from build123d import *

# Parameters (mm, degrees)
F1_DEPTH = 25
F3_DEPTH = 20


with BuildPart() as f1:
    # F0 (on Top) → F1 (new body)
    with BuildSketch(Plane.XY):
        with BuildLine():
            Line((-45.816002, -33.782002), (45.816002, -33.782002))
            ThreePointArc((45.816002, -33.782002), (50.058642, -32.024642), (51.816002, -27.782002))
            Line((51.816002, -27.782002), (51.816002, 27.782002))
            ThreePointArc((51.816002, 27.782002), (50.058642, 32.024642), (45.816002, 33.782002))
            Line((45.816002, 33.782002), (-45.816002, 33.782002))
            ThreePointArc((-45.816002, 33.782002), (-50.058642, 32.024642), (-51.816002, 27.782002))
            Line((-51.816002, 27.782002), (-51.816002, -27.782002))
            ThreePointArc((-51.816002, -27.782002), (-50.058642, -32.024642), (-45.816002, -33.782002))
        make_face()
    extrude(amount=F1_DEPTH)

    # F2 (on face) → F3 (cut)
    with BuildSketch(Plane.XY.offset(25)):
        with BuildLine():
            ThreePointArc((45.816002, -31.782002), (48.644429, -30.610429), (49.816002, -27.782002))
            Line((49.816002, -27.782002), (49.816002, 27.782002))
            ThreePointArc((49.816002, 27.782002), (48.644429, 30.610429), (45.816002, 31.782002))
            Line((45.816002, 31.782002), (-45.816002, 31.782002))
            ThreePointArc((-45.816002, 31.782002), (-48.644429, 30.610429), (-49.816002, 27.782002))
            Line((-49.816002, 27.782002), (-49.816002, -27.782002))
            ThreePointArc((-49.816002, -27.782002), (-48.644429, -30.610429), (-45.816002, -31.782002))
            Line((-45.816002, -31.782002), (45.816002, -31.782002))
        make_face()
    extrude(amount=-F3_DEPTH, mode=Mode.SUBTRACT)


solid = f1.part
Part model, mm, in its own coordinate system. A direction names the side the tool comes from. Round coordinates to 2 decimals unless told otherwise and drop trailing zeros. Loops run counter-clockwise (first coordinate to the right, second up) from the corner with the lowest first, then second, coordinate; pieces in that order, holes last. Notation, with made-up numbers: (-31.5, 60) - (-3.5, 60) arc R19 ccw to (-3.5, 78) - close; hole circle Ø7 at (47.5, 30.5). An arc over 180 degrees is marked (long way). Answer as a JSON object with one key per item and string values.
Item 1: Wall check: L1, parallel to X at y = 18, z = 11; L2, parallel to Y at x = 18, z = 22; L3, parallel to Z at x = 36, y = -14. Give the ranges that are in metal, low to high.
Output:
{"L1": "-51.82 to -49.82, 49.82 to 51.82", "L2": "-33.78 to -31.78, 31.78 to 33.78", "L3": "0 to 5"}
Item 2: Pin check, flat tip, straight feed: pin 1 (4 mm diameter, centred on x = 0, y = -18, fed in from +Z). Stop position of the tip, or through.
Output:
{"pin 1": "z = 5"}
Item 3: Pull direction X, two halves, no side cores. Call faces 1 (the face through (-48.675, -30.579, 15.14)), 2 (the face through (-1, -31.782, 15)), 3 (the face through (-50.105, -31.978, 12.325)), 4 (the face through (51.816, 0, 12)): pulls with the +X half, pulls with the -X half, needs draft (parallel to the pull), parting line crosses it, or undercut.
Output:
{"face 1": "undercut", "face 2": "undercut", "face 3": "pulls with the -X half", "face 4": "pulls with the +X half"}
Item 4: Band-saw the part on C-C on y = -6.5. List the corners of the cut face in (x, z).
Output:
{"outline": "(-51.82, 0) - (51.82, 0) - (51.82, 25) - (49.82, 25) - (49.82, 5) - (-49.82, 5) - (-49.82, 25) - (-51.82, 25) - close"}
Item 5: Band-saw the part on A-A on z = 20.25. List the corners of the cut face in (x, y).
Output:
{"outline": "(-51.82, -27.78) arc R6 ccw to (-45.82, -33.78) - (45.82, -33.78) arc R6 ccw to (51.82, -27.78) - (51.82, 27.78) arc R6 ccw to (45.82, 33.78) - (-45.82, 33.78) arc R6 ccw to (-51.82, 27.78) - close; hole (-49.82, -27.78) arc R4 ccw to (-45.82, -31.78) - (45.82, -31.78) arc R4 ccw to (49.82, -27.78) - (49.82, 27.78) arc R4 ccw to (45.82, 31.78) - (-45.82, 31.78) arc R4 ccw to (-49.82, 27.78) - close"}
Item 6: Band-saw the part on B-B on x = 24. List the corners of the cut face in (y, z), plus the area to 3 significant figures.
Output:
{"outline": "(-33.78, 0) - (33.78, 0) - (33.78, 25) - (31.78, 25) - (31.78, 5) - (-31.78, 5) - (-31.78, 25) - (-33.78, 25) - close", "area": "418 mm2"}
Item 7: Tool access for faces 5 (the face through (-49.816, 0, 15)), 6 (the face through (50.01, -32.07, 12.32)): list every direction of +Z, -Z, +X, -X, +Y, -Y with a clear straight run to the whole face (end or side of a thin tool).
Output:
{"face 5": "+Z", "face 6": "+Z, -Z, +X, -Y"}
